Read the model definition and answer for the solid it produces. Units are mm, in the model's axes. A direction names the side the tool comes from. Round coordinates to 2 decimals unless told otherwise and drop trailing zeros. Order: outer loops, then holes, each group sorted by start corner. A loop starts at its lowest first (then second) coordinate and runs counter-clockwise, first axis right, second up. Notation, with made-up numbers: (-24, 63.25) - (28, 63.25) arc R12 cw to (28, 77.25) - close; hole circle Ø3 at (29.25, 71.25). An arc over 180 degrees is marked (long way). Put each result on its own line as item: value. Start each with the question number.
Q1. Section A-A on z = -0.25 is taken. Give the vertices of the cut face in (x, y), then the cut area to 3 significant figures.
Q2. For a pull along Y with two mould halves and no side action, classify faces 1 (the face through (-3, 15, 12)), 2 (the face through (0, 28, 11)), 3 (the face through (-10, 11, 3)) as pulls with the +Y half, pulls with the -Y half, needs draft (parallel to the pull), parting line crosses it, or undercut.
Q3. Section B-B on x = 0 is taken. Give the vertices of the cut face in (y, z), then the cut area to 3 significant figures.
Q4. Section C-C on y = 14 is taken. Give the vertices of the cut face in (x, z).
Q5. Each of these flat-tipped pins is pushed along its axis until it touches: pin 1 Ø3.5 at (x, z) = (8, -10.5) entering from +Y; pin 2 Ø3.5 at (x, y) = (-9, 24.5) entering from -Z; pin 3 Ø5 at (x, z) = (-4, 6.5) entering from +Y. Where does it stop, or does it pass through?
Q6. Find the intervals of material crossed by line 1 along X through (y, z) = (12.5, 6.25); line 2 along Y through (x, z) = (3.5, -4.75); line 3 along Z through (x, y) = (8.5, 24), in increasing order. Write a range as from..to.
Q7. Which of the six approach directions +Z, -Z, +X, -X, +Y, -Y give full straight-line access (tool end or side, diameter ignored) to faces 4 (the face through (-2.4, 10.7, 14)), 5 (the face through (-9, 6.8, -11)), 6 (the face through (3, 2, -1)), 7 (the face through (3, 15, 12)), 8 (the face through (-7, 10, 4))?
Q8. Section D-D on y = 2.5 is taken. Give the vertices of the cut face in (x, z), then the cut area to 3 significant figures.
from build123d import *

# Parameters (mm, degrees)
SKETCH2_W           = 20
SKETCH2_H           = 28
BOSS_EXTRUDE1_DEPTH = 3.5
SKETCH3_W           = 20
SKETCH3_H           = 28
BOSS_EXTRUDE2_DEPTH = 3.5
BOSS_EXTRUDE3_DEPTH = 3
BOSS_EXTRUDE4_DEPTH = 3


with BuildPart() as part:
    # Sketch2 → Boss-Extrude1 (new body)
    with BuildSketch(Plane(origin=(0, 0, 0), x_dir=(1, 0, 0), z_dir=(0, 1, 0))):
        Rectangle(SKETCH2_W, SKETCH2_H)
        with BuildLine():
            Line((-3, -1), (-3, 3))
            ThreePointArc((-3, 3), (0, 6), (3, 3))
            Line((3, 3), (3, -1))
            ThreePointArc((3, -1), (0, -4), (-3, -1))
        make_face(mode=Mode.SUBTRACT)
    extrude(amount=BOSS_EXTRUDE1_DEPTH)

    # Sketch3 → Boss-Extrude2 (add)
    with BuildSketch(Plane.XY.offset(14)):
        with Locations((0, 14)):
            Rectangle(SKETCH3_W, SKETCH3_H)
        with BuildLine():
            Line((3, 17), (3, 13))
            ThreePointArc((3, 13), (0, 10), (-3, 13))
            Line((-3, 13), (-3, 17))
            ThreePointArc((-3, 17), (0, 20), (3, 17))
        make_face(mode=Mode.SUBTRACT)
    extrude(amount=-BOSS_EXTRUDE2_DEPTH)

    # Sketch4 → Boss-Extrude3 (add)
    with BuildSketch(Plane(origin=(10, 0, 0), x_dir=(0, 0, -1), z_dir=(1, 0, 0))):
        Polygon((-14, 0), (14, 0), (14, 6.8), (9, 6.8), (-7.2, 23), (-7.2, 28), (-14, 28), align=None)
    extrude(amount=-BOSS_EXTRUDE3_DEPTH)

    # Sketch5 → Boss-Extrude4 (add)
    with BuildSketch(Plane.ZY.offset(10)):
        Polygon((-14, 0), (14, 0), (14, 28), (7.2, 28), (7.2, 23), (-9, 6.8), (-14, 6.8), align=None)
    extrude(amount=-BOSS_EXTRUDE4_DEPTH)


solid = part.part
Findings:
1. outline: (-10, 0) - (-3, 0) - (-3, 3.5) - (-7, 3.5) - (-7, 15.55) - (-10, 15.55) - close; (3, 0) - (10, 0) - (10, 15.55) - (7, 15.55) - (7, 3.5) - (3, 3.5) - close
1. area: 121 mm2
2. face 1: undercut
2. face 2: pulls with the +Y half
2. face 3: needs draft
3. outline: (0, -14) - (3.5, -14) - (3.5, -6) - (0, -6) - close; (0, 4) - (3.5, 4) - (3.5, 10.5) - (10, 10.5) - (10, 14) - (0, 14) - close; (20, 10.5) - (28, 10.5) - (28, 14) - (20, 14) - close
3. area: 114 mm2
4. outline: (-10, -1.8) - (-7, -1.8) - (-7, 10.5) - (-3, 10.5) - (-3, 14) - (-10, 14) - close; (3, 10.5) - (7, 10.5) - (7, -1.8) - (10, -1.8) - (10, 14) - (3, 14) - close
5. pin 1: y = 7.05
5. pin 2: z = 6.95
5. pin 3: y = 3.5
6. line 1: -10..-7, 7..10
6. line 2: 0..3.5
6. line 3: 7.2..14
7. face 4: +Z, +X, -X, +Y, -Y
7. face 5: -Z, +X, -X, +Y
7. face 6: +Y, -Y
7. face 7: +Z, -Z
7. face 8: -Z, +Y
8. outline: (-10, -14) - (10, -14) - (10, 14) - (-10, 14) - close; hole (-3, -3) arc R3 ccw to (3, -3) - (3, 1) arc R3 ccw to (-3, 1) - close
8. area: 508 mm2
